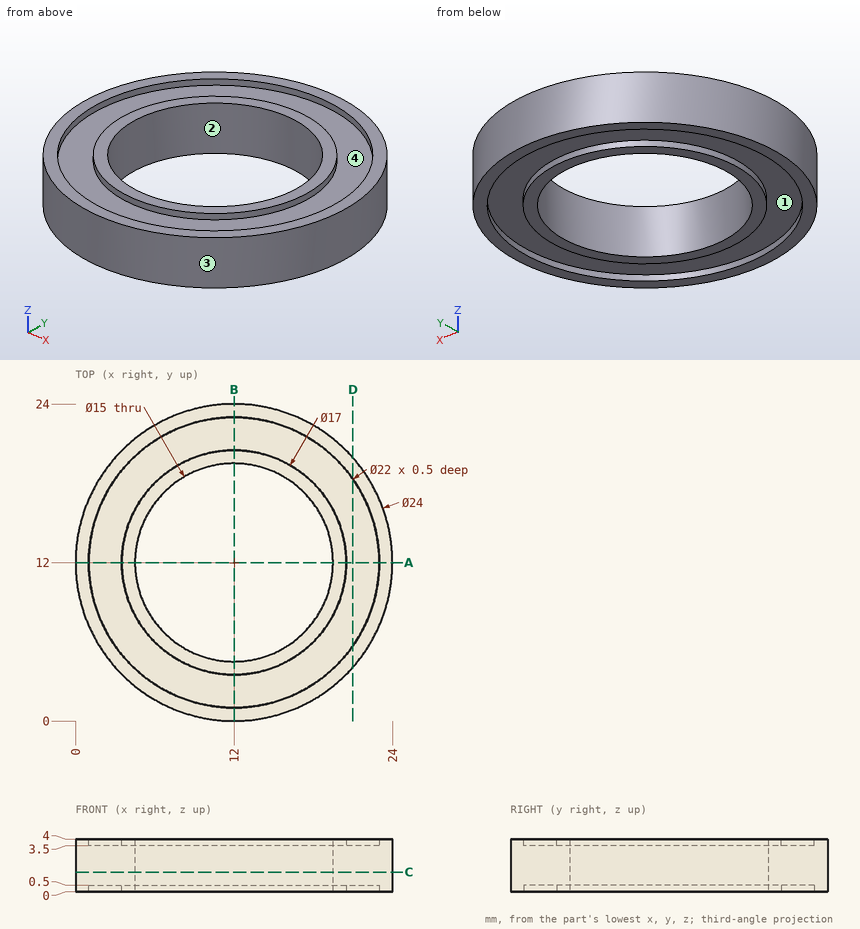
Could you check a few things on this drawing? It's one solid part, dimensions in mm from its lowest x, y, z. A direction names the side the tool comes from. Give positions to 0.01 mm unless a question says otherwise; leave off trailing zeros. Order: outer loops, then holes, each group sorted by start corner. A loop starts at its lowest first (then second) coordinate and runs counter-clockwise, first axis right, second up.
1. For pin 1 (1 mm diameter, centred on x = 3.5, z = 2, fed in from -Y), with a flat end and sliding along its axis, tell me the tip position at first contact or that it passes through.
Answers below:
pin 1: stops at y = 3.06
2. Which directions (+Z, -Z, +X, -X, +Y, -Y) give clear straight access to the entire face, cutting with the end or side of a thin tool? Please do the marked faces 1 and 2.
Answers below:
face 1: -Z
face 2: +Z, -Z
3. Suppose I cut it at D-D (x = 21). Write out the boundary of the cut face in (y, z), plus the area to 3 significant figures.
Answers below:
outline: (4.06, 0) - (5.68, 0) - (5.68, 0.5) - (18.32, 0.5) - (18.32, 0) - (19.94, 0) - (19.94, 4) - (18.32, 4) - (18.32, 3.5) - (5.68, 3.5) - (5.68, 4) - (4.06, 4) - close
area: 50.8 mm2
4. I need wall thicknesses on L1, parallel to Y at x = 12, z = 3.65; L2, parallel to Y at x = 13.5, z = 0.45; L3, parallel to Y at x = 12, z = 2.95. Which ranges of each line are inside material? Lowest first, please.
Answers below:
L1: y = 0 to 1, 3.5 to 4.5, 19.5 to 20.5, 23 to 24
L2: y = 0.09 to 1.1, 3.63 to 4.65, 19.35 to 20.37, 22.9 to 23.91
L3: y = 0 to 4.5, 19.5 to 24
5. Suppose I cut it at A-A (y = 12). Write out the boundary of the cut face in (x, z).
Answers below:
outline: (0, 0) - (1, 0) - (1, 0.5) - (3.5, 0.5) - (3.5, 0) - (4.5, 0) - (4.5, 4) - (3.5, 4) - (3.5, 3.5) - (1, 3.5) - (1, 4) - (0, 4) - close; (19.5, 0) - (20.5, 0) - (20.5, 0.5) - (23, 0.5) - (23, 0) - (24, 0) - (24, 4) - (23, 4) - (23, 3.5) - (20.5, 3.5) - (20.5, 4) - (19.5, 4) - close
6. Thinking about a two-plate mould opening in X: for the marked faces 3 and 4, which applies, +X half, -X half, draft (parallel to the pull), parting line (faces both ways), or undercut?
Answers below:
face 3: parting line
face 4: undercut
7. Suppose I cut it at C-C (z = 1.5). Write out the boundary of the cut face in (x, y), plus the area to 3 significant figures.
Answers below:
outline: circle Ø24 at (12, 12); hole circle Ø15 at (12, 12)
area: 276 mm2
